For this review, take the finished solid that the model builds, in its own axes (mm). Round coordinates to 2 decimals unless told otherwise and drop trailing zeros. Write each loop counter-clockwise with the first axis right and the second up, starting at its lowest first coordinate (ties: lowest second). Pieces come first, ordered by that corner, then holes. Notation, with made-up numbers: (38.5, 56.25) -> (76.5, 56.25) arc R36 ccw to (76.5, 93.25) -> close; hole circle Ø5 at (37.5, 22.5). An arc over 180 degrees is marked (long way). Answer as CSV lines item,"result". Start each with the question number.
Item 1: Take a section at D-D on z = -1. Give the boundary of the cut face in (x, y), then the cut area to 3 significant figures.
Item 2: Take a section at C-C on y = 6.5. Give the boundary of the cut face in (x, z), then the cut area to 3 significant figures.
Item 3: For pin 1 Ø3 at (y, z) = (2.5, -1.5) entering from -X; pin 2 Ø1 at (x, z) = (13.5, 1) entering from +Y; pin 3 Ø1.5 at (x, z) = (4, -1.5) entering from +Y; pin 4 Ø1.1 at (x, y) = (-11.26, 6.5) entering from +Z, all flat-tipped, find the tip position at first contact; note any pin that passes through.
Item 4: Take a section at B-B on x = 0. Give the boundary of the cut face in (y, z).
Item 5: Take a section at A-A on y = 13. Give the boundary of the cut face in (x, z).
Item 6: Wall thickness on probe 1 along Y at (x, z) = (0, 0.05); probe 2 along Y at (x, z) = (-10.5, 0.15); probe 3 along X at (y, z) = (7, 0.65): over which ranges is each line inside the solid? List them lowest first. Write a range as from..to.
```python
from build123d import *

# Parameters (mm, degrees)
SKETCH_1_R               = 18.5
SKETCH_1_R_2             = 1.1
EXTRUDE_1_DEPTH          = 2.5
SKETCH_2_R               = 0.9
CUT_EXTRUDE_1_DEPTH      = 27.636441204
PATTERN_CIRCULAR_1_COUNT = 6


with BuildPart() as part:
    # 草图1 → 凸台-拉伸1 (new, symmetric)
    with BuildSketch(Plane.XY):
        Circle(SKETCH_1_R)
        Circle(SKETCH_1_R_2, mode=Mode.SUBTRACT)
    extrude(amount=EXTRUDE_1_DEPTH, both=True)

    # 草图2 → 切除-拉伸1 (cut, through all)
    with BuildSketch(Plane.XY.offset(2.5)):
        with Locations((0, 13)):
            Circle(SKETCH_2_R)
    cut_extrude_1 = extrude(amount=-CUT_EXTRUDE_1_DEPTH, mode=Mode.SUBTRACT)

    # 阵列(圆周)1: 切除-拉伸1 ×6 about axis
    pattern_circular_1_axis = Axis((0, 0, 0), (0, 0, 1))
    for i in range(1, PATTERN_CIRCULAR_1_COUNT):
        add(cut_extrude_1.rotate(pattern_circular_1_axis, i * 360 / PATTERN_CIRCULAR_1_COUNT), mode=Mode.SUBTRACT)


solid = part.part
```
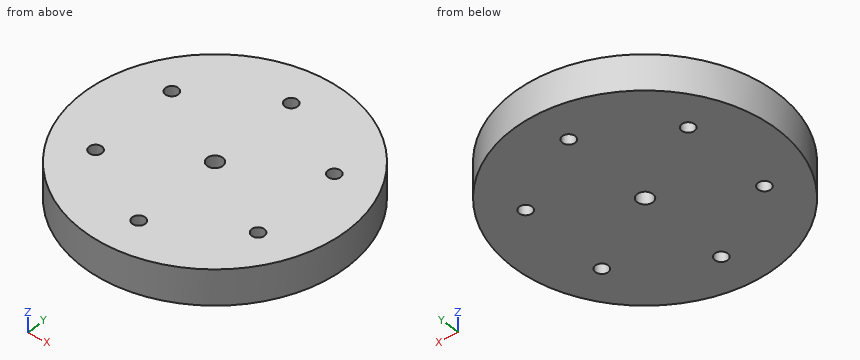
Output values:
1,outline,"circle Ø37 at (0, 0); hole circle Ø1.8 at (-11.26, -6.5); hole circle Ø1.8 at (-11.26, 6.5); hole circle Ø2.2 at (0, 0); hole circle Ø1.8 at (0, -13); hole circle Ø1.8 at (0, 13); hole circle Ø1.8 at (11.26, -6.5); hole circle Ø1.8 at (11.26, 6.5)"
1,area,"1,060 mm^2"
2,outline,"(-17.32, -2.5) -> (-12.16, -2.5) -> (-12.16, 2.5) -> (-17.32, 2.5) -> close; (-10.36, -2.5) -> (10.36, -2.5) -> (10.36, 2.5) -> (-10.36, 2.5) -> close; (12.16, -2.5) -> (17.32, -2.5) -> (17.32, 2.5) -> (12.16, 2.5) -> close"
2,area,"155 mm^2"
3,pin 1,"stops at x = -18.47"
3,pin 2,"stops at y = 13.16"
3,pin 3,"stops at y = 18.21"
3,pin 4,"passes through"
4,outline,"(-18.5, -2.5) -> (-13.9, -2.5) -> (-13.9, 2.5) -> (-18.5, 2.5) -> close; (-12.1, -2.5) -> (-1.1, -2.5) -> (-1.1, 2.5) -> (-12.1, 2.5) -> close; (1.1, -2.5) -> (12.1, -2.5) -> (12.1, 2.5) -> (1.1, 2.5) -> close; (13.9, -2.5) -> (18.5, -2.5) -> (18.5, 2.5) -> (13.9, 2.5) -> close"
5,outline,"(-13.16, -2.5) -> (-0.9, -2.5) -> (-0.9, 2.5) -> (-13.16, 2.5) -> close; (0.9, -2.5) -> (13.16, -2.5) -> (13.16, 2.5) -> (0.9, 2.5) -> close"
6,probe 1,"y = -18.5..-13.9, -12.1..-1.1, 1.1..12.1, 13.9..18.5"
6,probe 2,"y = -15.23..-6.98, -6.02..6.02, 6.98..15.23"
6,probe 3,"x = -17.12..-12.01, -10.51..10.51, 12.01..17.12"
